Geometry check sheet. Reference: drawing and pictorial views, mm from the part's lowest x, y, z. A direction names the side the tool comes from. Coordinates: 2 decimals unless noted, no trailing zeros. Order: outer loops, then holes, each group sorted by start corner. A loop starts at its lowest first (then second) coordinate and runs counter-clockwise, first axis right, second up. Notation, with made-up numbers: M 59.25,57 L 66.25,57 A24 cw 66.25,81 Z; hole C 73,59 d10. An arc over 180 degrees is marked long. Return JSON: item names as keys, results as strings.
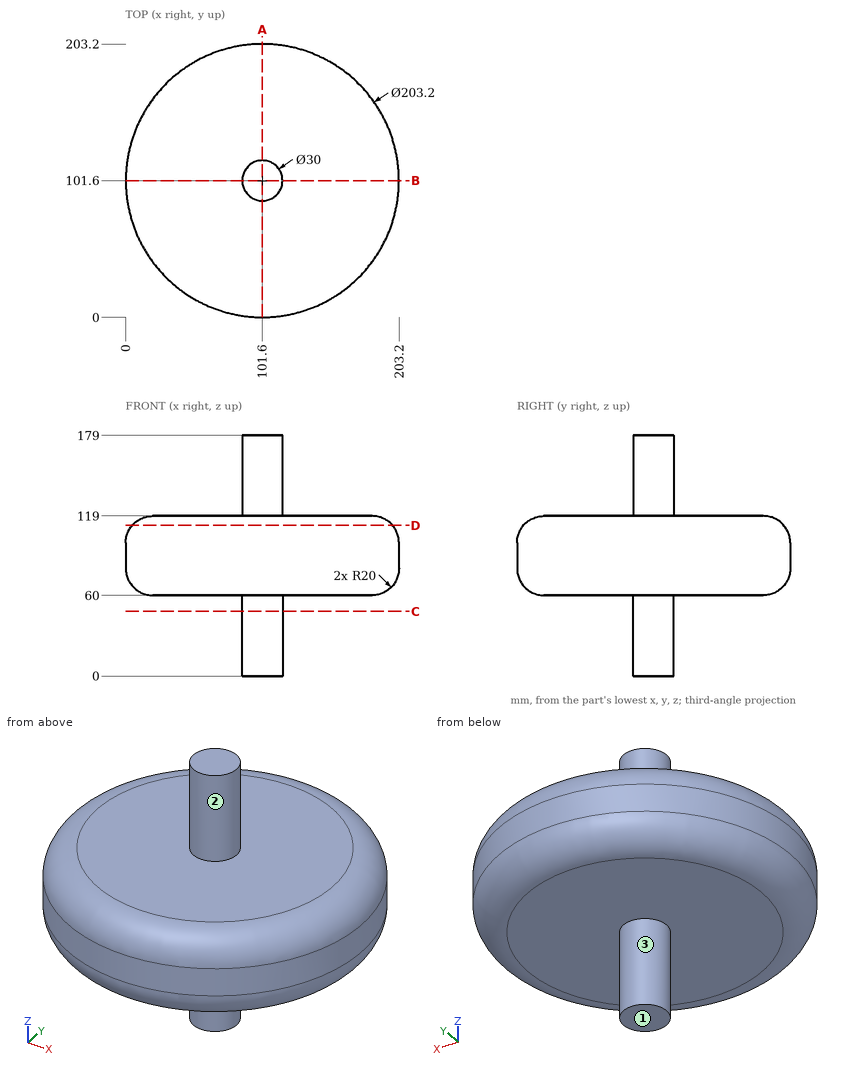
Q1. Tool access check on the marked faces 1, 2 and 3. Record the directions out of +Z, -Z, +X, -X, +Y, -Y that give a thin tool (end or side, any length) a straight path to the whole face; none if there is none.
Values:
{"face 1": "-Z, +X, -X, +Y, -Y", "face 2": "+Z", "face 3": "-Z"}
Q2. Cross-section at C-C, the plane z = 48. Record the boundary of the cut face in (x, y).
Values:
{"outline": "C 101.6,101.6 d30"}
Q3. Cross-section at A-A, the plane x = 101.6. Record the boundary of the cut face in (y, z).
Values:
{"outline": "M 0,80 A20 ccw 20,60 L 86.6,60 L 86.6,0 L 116.6,0 L 116.6,60 L 183.2,60 A20 ccw 203.2,80 L 203.2,99 A20 ccw 183.2,119 L 116.6,119 L 116.6,179 L 86.6,179 L 86.6,119 L 20,119 A20 ccw 0,99 Z"}
Q4. Go/stop test with flat-tipped pins: pin 1 (6 mm diameter, centred on x = 88, z = 61.5, fed in from +Y); pin 2 (6 mm diameter, centred on x = 180.5, z = 68, fed in from +Y); pin 3 (2 mm diameter, centred on x = 179.5, y = 113.5, fed in from +Z); pin 4 (6 mm diameter, centred on x = 104.5, y = 85.5, fed in from -Z). Record where each tip stops, or that it passes through.
Values:
{"pin 1": "y = 194.88", "pin 2": "y = 164.13", "pin 3": "z = 119", "pin 4": "z = 0"}
Q5. Cross-section at D-D, the plane z = 112. Record the boundary of the cut face in (x, y).
Values:
{"outline": "C 101.6,101.6 d193.6"}
Q6. Material ranges on line 1 along Z through (x, y) = (128, 25); line 2 along X through (y, z) = (102.5, 130.5); line 3 along Z through (x, y) = (28.5, 147), recorded low to high.
Values:
{"line 1": "60 to 119", "line 2": "86.63 to 116.57", "line 3": "60.5 to 118.5"}
